Geometry check sheet. Reference: drawing and pictorial views, mm from the part's lowest x, y, z. A direction names the side the tool comes from. Round coordinates to 2 decimals unless told otherwise and drop trailing zeros. Order: outer loops, then holes, each group sorted by start corner. A loop starts at its lowest first (then second) coordinate and runs counter-clockwise, first axis right, second up.
(1) Gauge pin test, flat ends, axial feed: P1, Ø10, axis at y = 82, z = 22, coming from the -X side; P2, Ø6, axis at y = 21.5, z = 102.5, coming from the +X side; P3, Ø5, axis at x = 24.5, y = 106, coming from the -Z side. Record the tip position at first contact, or that the pin passes through.
(2) Set-up check for the marked faces 1, 2 and 3: record each of +Z, -Z, +X, -X, +Y, -Y from which the full face is reachable in a straight line by a thin tool's end or side.
(3) Cross-section at A-A on x = 18. Enter the section's corners in (y, z) (1 decimal), and give its area (3 significant figures).
(4) Thickness scan on L1, parallel to X at y = 155.5, z = 79; L2, parallel to Z at x = 25.75, y = 68; L3, parallel to Y at x = 18.5, z = 67 (1 decimal). Record the ranges inside material, lowest first.
(5) Cross-section at D-D on y = 121. Enter the section's corners in (x, z), and give its area (3 significant figures).
(6) Cross-section at C-C on z = 94.5. Enter the section's corners in (x, y).
(7) Cross-section at B-B on y = 74. Enter the section's corners in (x, z).
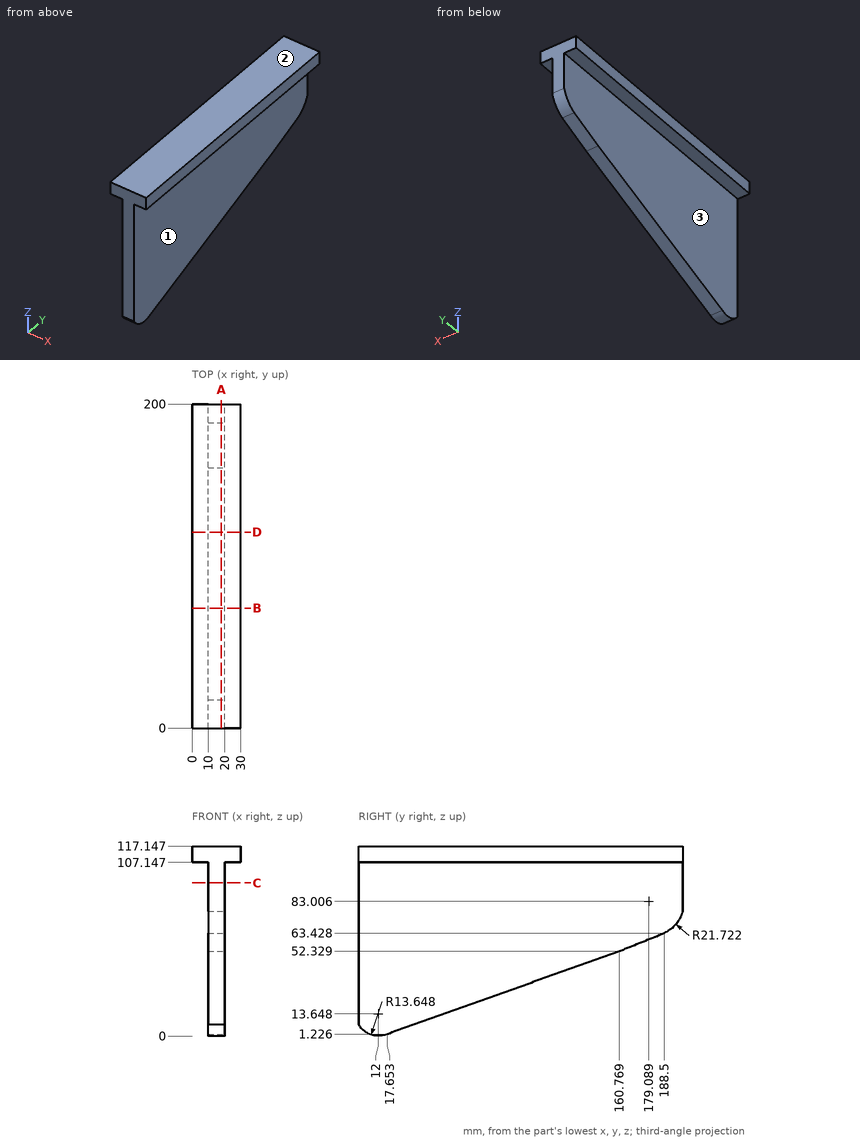
Found:
1. P1: stops at x = 10
1. P2: stops at x = 20
1. P3: stops at z = 107.15
2. face 1: -Z, +X, +Y, -Y
2. face 2: +Z, +X, -X, +Y, -Y
2. face 3: -Z, -X, +Y, -Y
3. outline: (0, 7.1) arc R13.6 ccw to (17.7, 1.2) - (160.8, 52.3) - (188.5, 63.4) arc R21.7 ccw to (200, 77.1) - (200, 117.1) - (0, 117.1) - close
3. area: 17,200 mm2
4. L1: x = 10 to 20
4. L2: z = 107.15 to 117.15
4. L3: y = 0 to 193.8
5. outline: (0, 107.15) - (10, 107.15) - (10, 38.13) - (20, 38.13) - (20, 107.15) - (30, 107.15) - (30, 117.15) - (0, 117.15) - close
5. area: 990 mm2
6. outline: (10, 0) - (20, 0) - (20, 200) - (10, 200) - close
7. outline: (0, 107.15) - (10, 107.15) - (10, 21.35) - (20, 21.35) - (20, 107.15) - (30, 107.15) - (30, 117.15) - (0, 117.15) - close
